from build123d import *

# Parameters (mm, degrees)
SKETCH1_R           = 1.5
BOSS_EXTRUDE1_DEPTH = 5
SKETCH2_W           = 30
SKETCH2_H           = 2.5
BOSS_EXTRUDE2_DEPTH = 26
FILLET1_R           = 13
CUT_EXTRUDE1_START  = -13
CUT_EXTRUDE1_DEPTH  = 52.939054945
SKETCH4_R           = 7.6
CUT_EXTRUDE2_DEPTH  = 1.2
SKETCH5_R           = 6.6
CUT_EXTRUDE3_DEPTH  = 47.080312024
CUT_EXTRUDE4_START  = 1.2
SKETCH6_R           = 7.6
CUT_EXTRUDE4_DEPTH  = 1.2
SKETCH7_R           = 6.6
CUT_EXTRUDE5_DEPTH  = 47.080312024
SKETCH8_R           = 4
CUT_EXTRUDE6_DEPTH  = 47.080312024


with BuildPart() as part:
    # Sketch1 → Boss-Extrude1 (new body)
    with BuildSketch(Plane(origin=(0, 0, 0), x_dir=(1, 0, 0), z_dir=(0, 1, 0))):
        Polygon((0, 0), (6, 0), (6, -10), (20, -10), (20, 0), (26, 0), (26, -10), (28, -10), (28, -36), (-2, -36), (-2, -10), (0, -10), align=None)
        with Locations(Location((3, -5, 0), (0, 0, 270))):
            Circle(SKETCH1_R, mode=Mode.SUBTRACT)
        with Locations(Location((23, -5, 0), (0, 0, 90))):
            Circle(SKETCH1_R, mode=Mode.SUBTRACT)
    extrude(amount=BOSS_EXTRUDE1_DEPTH)

    # Sketch2 → Boss-Extrude2 (add)
    with BuildSketch(Plane.XY.offset(36)):
        with Locations((13, 6.25)):
            Rectangle(SKETCH2_W, SKETCH2_H)
        with Locations((13, -1.25)):
            Rectangle(SKETCH2_W, SKETCH2_H)
    extrude(amount=-BOSS_EXTRUDE2_DEPTH)

    # Fillet1
    fillet1_edges = [part.edges().sort_by_distance(p)[0] for p in [
        (28, 2.5, 36),
        (-2, 2.5, 36),
    ]]
    fillet(fillet1_edges, radius=FILLET1_R)

    # Sketch3 → Cut-Extrude1 (cut)
    with BuildSketch(Plane(origin=(0, 0, 10), x_dir=(-1, 0, 0), z_dir=(0, 0, -1)).offset(CUT_EXTRUDE1_START)):
        Polygon((-19.6, 7.5), (-19.6, 5.2875), (-20.6, 5.2875), (-20.6, 4.0875), (-13, 4.0875), (-5.4, 4.0875), (-5.4, 5.2875), (-6.4, 5.2875), (-6.4, 7.5), align=None)
    cut_extrude1 = extrude(amount=CUT_EXTRUDE1_DEPTH, mode=Mode.SUBTRACT)

    # Sketch4 → Cut-Extrude2 (cut)
    with BuildSketch(Plane(origin=(0, 4.0875, 0), x_dir=(1, 0, 0), z_dir=(0, 1, 0))):
        with Locations((13, -23)):
            Circle(SKETCH4_R)
    extrude(amount=CUT_EXTRUDE2_DEPTH, mode=Mode.SUBTRACT)

    # Sketch5 → Cut-Extrude3 (cut, through all)
    with BuildSketch(Plane(origin=(0, 4.0875, 0), x_dir=(1, 0, 0), z_dir=(0, 1, 0))):
        with Locations((13, -23)):
            Circle(SKETCH5_R)
    extrude(amount=CUT_EXTRUDE3_DEPTH, mode=Mode.SUBTRACT)

    # Mirror1: Cut-Extrude1 across plane
    add(cut_extrude1.mirror(Plane(origin=(0, 2.5, 0), x_dir=(0, 0, 1), z_dir=(0, -1, 0))), mode=Mode.SUBTRACT)

    # Sketch6 → Cut-Extrude4 (cut)
    with BuildSketch(Plane.XZ.offset(-0.9125).offset(CUT_EXTRUDE4_START)):
        with Locations((13, 23)):
            Circle(SKETCH6_R)
    extrude(amount=-CUT_EXTRUDE4_DEPTH, mode=Mode.SUBTRACT)

    # Sketch7 → Cut-Extrude5 (cut, through all)
    with BuildSketch(Plane.XZ.offset(-0.9125)):
        with Locations((13, 23)):
            Circle(SKETCH7_R)
    extrude(amount=CUT_EXTRUDE5_DEPTH, mode=Mode.SUBTRACT)

    # Sketch8 → Cut-Extrude6 (cut, through all)
    with BuildSketch(Plane(origin=(0, 4.0875, 0), x_dir=(1, 0, 0), z_dir=(0, 1, 0))):
        with Locations(Location((13, -23, 0), (0, 0, 270))):
            Circle(SKETCH8_R)
    extrude(amount=-CUT_EXTRUDE6_DEPTH, mode=Mode.SUBTRACT)


solid = part.part
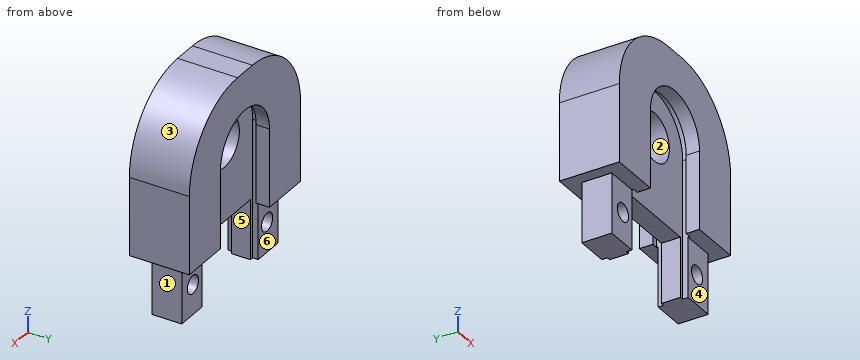
Source: CAD feature listing. Evaluate the final solid. Frame: model axes, mm. Face numbers are marked on the shaded views. A direction names the side the tool comes from. Coordinates: 2 decimals unless noted, no trailing zeros. Loops run counter-clockwise (first coordinate to the right, second up) from the corner with the lowest first, then second, coordinate; pieces in that order, holes last. Notation, with made-up numbers: (88, 70.25) -> (102, 70.25) arc R29 ccw to (102, 102.25) -> close; hole circle Ø6 at (83.5, 69.5). An arc over 180 degrees is marked (long way). Answer in a Markdown table with one row per item. Add a question column.
Q1. Section B-B on z = 5. Return the cut outline in (x, y).
Q2. Section C-C on y = 2. Return the cut outline in (x, z), and give its area (3 significant figures).
Q3. Ray query, line 1 along X through (y, z) = (1.7, 5); line 2 along X through (y, z) = (3, 2); line 3 along X through (y, z) = (2.8, 23). Return the intervals inside material, ascending.
Q4. Reachability of the marked faces 4, 5 and 6 from +Z, -Z, +X, -X, +Y, -Y: full face, straight path, thin tool, end or side. Return the list, or none.
Q5. Contact query for flat-ended pins moving along their axis: pin 1 Ø2 at (x, y) = (6, 0) entering from +Z; pin 2 Ø6 at (y, z) = (6.5, 32) entering from -X; pin 3 Ø4.5 at (x, z) = (14.5, 9.5) entering from -Y; pin 4 Ø2.5 at (x, z) = (23, 5) entering from +Y. Output: stop coordinate, or through.
Q6. Section D-D on z = 17. Return the cut outline in (x, y), and give its area (3 significant figures).
Q7. Pull-direction query (Z, two-part tool) for the marked faces 1, 2 and 3; classes: pulls with the +Z half, pulls with the -Z half, needs draft (parallel to the pull), parting line crosses it, or undercut.
Q8. Section A-A on x = 13. Return the cut outline in (y, z), and give its area (3 significant figures).
Computed values:
| question | item | result |
|---|---|---|
| 1 | outline | (0, 0) -> (1.5, 0) -> (1.5, 5) -> (0, 5) -> close; (4.5, 0) -> (5.4, 0) -> (5.4, 0.91) -> (6, 0.91) -> (6, 4.09) -> (5.4, 4.09) -> (5.4, 5) -> (4.5, 5) -> close; (20, 0.91) -> (20.6, 0.91) -> (20.6, 0) -> (21.5, 0) -> (21.5, 5) -> (20.6, 5) -> (20.6, 4.09) -> (20, 4.09) -> close; (24.5, 0) -> (26, 0) -> (26, 5) -> (24.5, 5) -> close |
| 2 | outline | (-2, 10) -> (0, 10) -> (0, 0) -> (6, 0) -> (6, 10) -> (20, 10) -> (20, 0) -> (26, 0) -> (26, 10) -> (28, 10) -> (28, 23) arc R13 ccw to (15, 36) -> (11, 36) arc R13 ccw to (-2, 23) -> close; hole circle Ø3 at (3, 5); hole circle Ø8 at (13, 23); hole circle Ø3 at (23, 5) |
| 2 | area | 763 mm^2 |
| 3 | line 1 | x = 0 to 1.5, 4.5 to 6, 20 to 21.5, 24.5 to 26 |
| 3 | line 2 | x = 0 to 6, 20 to 26 |
| 3 | line 3 | x = -2 to 9, 17 to 28 |
| 4 | face 4 | -Z, +X, -X, -Y |
| 4 | face 5 | -Z, +Y, -Y |
| 4 | face 6 | -Z, +X, -X, +Y |
| 5 | pin 1 | stops at z = 35.37 |
| 5 | pin 2 | stops at x = -0.53 |
| 5 | pin 3 | stops at y = 0.91 |
| 5 | pin 4 | passes through |
| 6 | outline | (-2, -2.5) -> (6.4, -2.5) -> (6.4, -0.29) -> (5.4, -0.29) -> (5.4, 0.91) -> (20.6, 0.91) -> (20.6, -0.29) -> (19.6, -0.29) -> (19.6, -2.5) -> (28, -2.5) -> (28, 7.5) -> (19.6, 7.5) -> (19.6, 5.29) -> (20.6, 5.29) -> (20.6, 4.09) -> (5.4, 4.09) -> (5.4, 5.29) -> (6.4, 5.29) -> (6.4, 7.5) -> (-2, 7.5) -> close |
| 6 | area | 205 mm^2 |
| 7 | face 1 | needs draft |
| 7 | face 2 | undercut |
| 7 | face 3 | pulls with the +Z half |
| 8 | outline | (-2.5, 29.6) -> (-0.29, 29.6) -> (-0.29, 30.6) -> (0.91, 30.6) -> (0.91, 27) -> (4.09, 27) -> (4.09, 30.6) -> (5.29, 30.6) -> (5.29, 29.6) -> (7.5, 29.6) -> (7.5, 36) -> (-2.5, 36) -> close; (0.91, 10) -> (4.09, 10) -> (4.09, 19) -> (0.91, 19) -> close |
| 8 | area | 98.4 mm^2 |
